Autodesk Inventor part; units mm, degrees
ref_plane "YZ Plane" through (0, 0, 0) normal (1, 0, 0) x (0, 1, 0)
ref_plane "XZ Plane" through (0, 0, 0) normal (0, 1, 0) x (-1, 0, 0)
ref_plane "XY Plane" through (0, 0, 0) normal (0, 0, 1) x (1, 0, 0)
sketch "Sketch1" plane through (0, 0, 0) normal (0, 0, 1) x (1, 0, 0)
  line L0 (-9.1129, 4.4946) -> (-3.1129, 4.4946)
  line L1 (-3.1129, 4.4946) -> (-3.1129, -3.7524)
  line L2 (-3.1129, -3.7524) -> (-9.1129, -3.7524)
  line L3 (-9.1129, -3.7524) -> (-9.1129, 4.4946)
  line L4 (-9.1129, 4.4946) -> (-7.1129, 4.4946)
  line L5 (-7.1129, 4.4946) -> (-7.1129, -3.7524)
  line L6 (-7.1129, -3.7524) -> (-9.1129, -3.7524)
  line L7 (-9.1129, -3.7524) -> (-9.1129, 4.4946)
  line L8 (-3.1129, 4.4946) -> (-5.1129, 4.4946)
  line L9 (-5.1129, 4.4946) -> (-5.1129, -3.7524)
  line L10 (-5.1129, -3.7524) -> (-3.1129, -3.7524)
  line L11 (-3.1129, -3.7524) -> (-3.1129, 4.4946)
  point P0 (0, 0)
  dimension "d0" = 6
  dimension "d1" = 2
  dimension "d2" = 2
extrude "Extrusion1" add sketch "Sketch1" along normal blind 5 contours L0 L5 L2 L3 | L0 L1 L2 L9
sketch "Sketch2" plane through (0, 0, 5) normal (0, 0, 1) x (1, 0, 0)
  line L0 (-9.1129, 4.4946) -> (-3.1129, 4.4946)
  line L1 (-3.1129, 4.4946) -> (-3.1129, -3.7524)
  line L2 (-3.1129, -3.7524) -> (-9.1129, -3.7524)
  line L3 (-9.1129, -3.7524) -> (-9.1129, 4.4946)
  point P0 (0, 0)
extrude "Extrusion2" add sketch "Sketch2" against normal blind 2
properties part number "Roller ver2"
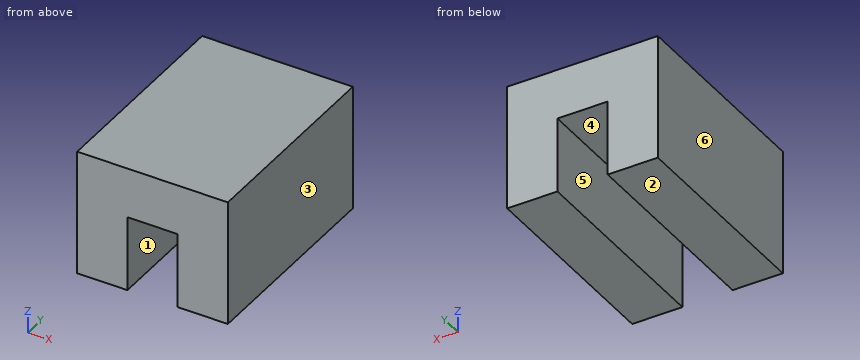
For this review, take the finished solid that the model builds, in its own axes (mm). Face numbers are marked on the shaded views. A direction names the side the tool comes from. Round coordinates to 2 decimals unless told otherwise and drop trailing zeros. Order: outer loops, then holes, each group sorted by start corner. A loop starts at its lowest first (then second) coordinate and runs counter-clockwise, first axis right, second up. Notation, with made-up numbers: (-5.75, -2.5) -> (43.25, -2.5) arc R29 ccw to (43.25, 26.5) -> close; hole circle Ø10 at (24.5, 36.5). An arc over 180 degrees is marked (long way). Write item = value, one per line. Start each with the question number.
1) The part is to be moulded in two halves that separate along X. For the marked faces 1, 2, 3 and 4, say which applies: +X half, -X half, draft (parallel to the pull), parting line (faces both ways), or undercut.
2) Tool access review of the marked faces 5 and 6: name each direction out of +Z, -Z, +X, -X, +Y, -Y from which nothing blocks a thin tool from reaching the whole face with its end or side.
3) Take a section at C-C on x = -6.25. State the section outline as (y, z) points, plus the area to 3 significant figures.
4) Take a section at B-B on y = 2. State the section outline as (x, z) points, plus the area to 3 significant figures.
5) To check wall thickness, follow line 1 (X direction, y = -1.25, z = 2.9); line 2 (Z direction, x = -5.7, y = 3.25). State the ranges of each line that lie inside material, in increasing order. Write a range as from..to.
6) Take a section at A-A on z = 1.85. State the section outline as (x, y) points.
Verdict:
q1.face_1 = undercut
q1.face_2 = draft
q1.face_3 = +X half
q1.face_4 = undercut
q2.face_5 = -Z, +Y, -Y
q2.face_6 = +Z, -Z, -X, +Y, -Y
q3.outline = (-3.75, 3) -> (4.49, 3) -> (4.49, 5) -> (-3.75, 5) -> close
q3.area = 16.5 mm2
q4.outline = (-9.11, 0) -> (-7.11, 0) -> (-7.11, 3) -> (-5.11, 3) -> (-5.11, 0) -> (-3.11, 0) -> (-3.11, 5) -> (-9.11, 5) -> close
q4.area = 24.0 mm2
q5.line_1 = -9.11..-7.11, -5.11..-3.11
q5.line_2 = 3..5
q6.outline = (-9.11, -3.75) -> (-7.11, -3.75) -> (-7.11, 4.49) -> (-9.11, 4.49) -> close; (-5.11, -3.75) -> (-3.11, -3.75) -> (-3.11, 4.49) -> (-5.11, 4.49) -> close
